Autodesk Inventor part; units mm, degrees
ref_plane "YZ Plane" through (0, 0, 0) normal (1, 0, 0) x (0, 1, 0)
ref_plane "XZ Plane" through (0, 0, 0) normal (0, 1, 0) x (-1, 0, 0)
ref_plane "XY Plane" through (0, 0, 0) normal (0, 0, 1) x (1, 0, 0)
sketch "Skizze2" plane through (0, 0, 0) normal (0, 0, 1) x (1, 0, 0)
  line L0 (-26.1954, 0) -> (26.1954, 0)
  line L1 (0, -30.2532) -> (0, 68.0422)
  line L2 (-18.5, 54) -> (-18.5, -6.7574)
  line L3 (-9.2574, -16) -> (9.2574, -16)
  line L4 (18.5, -6.7574) -> (18.5, 54)
  line L5 (18.5, 54) -> (11, 54)
  line L6 (11, 54) -> (11, 3)
  line L7 (-11, 3) -> (-11, 54)
  line L8 (-11, 54) -> (-18.5, 54)
  circle A0 centre (0, -10) radius 3.15
  circle A1 centre (-14.75, 43) radius 1.3
  circle A2 centre (-14.75, 30) radius 1.3
  circle A3 centre (-14.75, 17) radius 1.3
  circle A4 centre (-14.75, 3) radius 1.3
  circle A5 centre (14.75, 43) radius 1.3
  circle A6 centre (14.75, 30) radius 1.3
  circle A7 centre (14.75, 17) radius 1.3
  circle A8 centre (14.75, 3) radius 1.3
  line L9 (-17.6213, -8.8787) -> (-11.3787, -15.1213)
  line L10 (11.3787, -15.1213) -> (17.6213, -8.8787)
  arc A9 (-18.5, -6.7574) -> (-17.6213, -8.8787) centre (-15.5, -6.7574) ccw
  arc A10 (-11.3787, -15.1213) -> (-9.2574, -16) centre (-9.2574, -13) ccw
  arc A11 (9.2574, -16) -> (11.3787, -15.1213) centre (9.2574, -13) ccw
  line L11 (-11, 3) -> (-11, 0.2426)
  line L12 (11, 3) -> (11, 0.2426)
  line L13 (-6.7574, -4) -> (6.7574, -4)
  line L14 (-10.1213, -1.8787) -> (-8.8787, -3.1213)
  line L15 (8.8787, -3.1213) -> (10.1213, -1.8787)
  arc A12 (-11, 0.2426) -> (-10.1213, -1.8787) centre (-8, 0.2426) ccw
  arc A13 (-8.8787, -3.1213) -> (-6.7574, -4) centre (-6.7574, -1) ccw
  arc A14 (6.7574, -4) -> (8.8787, -3.1213) centre (6.7574, -1) ccw
  arc A15 (10.1213, -1.8787) -> (11, 0.2426) centre (8, 0.2426) ccw
  arc A16 (17.6213, -8.8787) -> (18.5, -6.7574) centre (15.5, -6.7574) ccw
  point P0 (0, 0)
  point P1 (-18.5, -16)
  point P2 (18.5, -16)
  point P3 (11, 0)
  point P4 (-11, 0)
  point P5 (-8, 0)
  point P6 (-11, 3)
  point P7 (8, 0)
  point P8 (11, 3)
  point P9 (-18.5, -8)
  point P10 (-10.5, -16)
  point P11 (10.5, -16)
  point P12 (18.5, -8)
  point P13 (-11, -4)
  point P14 (11, -4)
  point P15 (-11, -1)
  point P16 (-8, -4)
  point P17 (8, -4)
  point P18 (11, -1)
  dimension "d0" = 70
  dimension "d1" = 37
  dimension "d2" = 90
  dimension "d3" = 70
  dimension "d4" = 90
  dimension "d6" = 7.5
  dimension "d8" = 90
  dimension "d9" = 22
  dimension "d10" = 54
  dimension "d11" = 6.3
  dimension "d13" = 6
  dimension "d14" = 2.6
  dimension "d15" = 3.75
  dimension "d16" = 11
  dimension "d17" = 2.6
  dimension "d18" = 2.6
  dimension "d19" = 2.6
  dimension "d20" = 13
  dimension "d21" = 13
  dimension "d22" = 14
  dimension "d23" = 3.75
  dimension "d24" = 3.75
  dimension "d25" = 3.75
  dimension "d26" = 2.6
  dimension "d27" = 2.6
  dimension "d28" = 2.6
  dimension "d29" = 2.6
  dimension "d30" = 3.75
  dimension "d31" = 3
  dimension "d32" = 3
  dimension "d33" = 3
  dimension "d34" = 3
  dimension "d35" = 8
  dimension "d36" = 8
  dimension "d37" = 8
  dimension "d38" = 8
  dimension "d45" = 7
  dimension "d46" = 7
  dimension "d47" = 3
  dimension "d48" = 3
  dimension "d49" = 3
  dimension "d50" = 3
  dimension "d51" = 3
  dimension "d52" = 90
  dimension "d53" = 54
  dimension "d54" = 4
  dimension "d55" = 11
  dimension "d56" = 8
  dimension "d57" = 8
  dimension "d58" = 3
extrude "Extrusion1" add sketch "Skizze2" along normal blind 4 contours L2 L8 L7 L11 A12 L0 | L0 A12 L14 A13 L13 L1 A0 L3 A10 L9 A9 L2 | A15 L12 L6 L5 L4 L0 | L0 L4 A16 L10 A11 L3 L1 A0 L13 A14 L15 A15
equation "\"d14\" = d29"
equation "\"d17\" = d28"
equation "\"d18\" = d28"
equation "\"d19\" = d29"
equation "\"d23\" = d24"
equation "\"d24\" = d25"
equation "\"d25\" = d15"
equation "\"d26\" = d29"
equation "\"d27\" = d28"
equation "\"d28\" = d29"
equation "\"d30\" = d15"
properties part number "Part1_new1" material "Aluminium 6061"
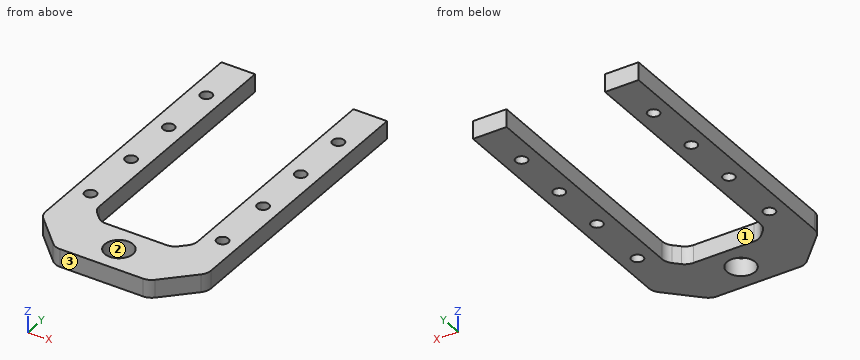
Model file for the job. Use its own axes, mm. Face numbers are marked on the shaded views. Give positions to 0.01 mm unless a question says otherwise; leave off trailing zeros. Loops run counter-clockwise (first coordinate to the right, second up) from the corner with the lowest first, then second, coordinate; pieces in that order, holes last.
1) Saw through at B-B (y = 43). Write the cut outline in (x, z).
2) Saw through at A-A (x = 0). Write the cut outline in (y, z).
3) Saw through at D-D (x = -14.75). Write the cut outline in (y, z).
4) Wall check: line 1 (X direction, y = 9.5, z = 1.2); line 2 (Y direction, x = -14.75, z = 2.4); line 3 (Y direction, x = 0, z = 0.45). Give the ranges that are in metal, low to high.
5) Flat gauge pin, fed straight in: pin 1 Ø1 at (x, z) = (-11.5, 3.5) entering from -Y. Where does the tip first touch, or does it go through?
6) Pull direction Y, two halves, no side cores. Call the marked faces 1, 2 and 3: +Y half, -Y half, draft (parallel to the pull), parting line (faces both ways), or undercut.
7) Saw through at C-C (z = 1.8). Count the separate pieces of the cut face and the enclosed holes in it, plus the area to 3 significant figures.
Answer block:
1. outline: (-18.5, 0) - (-16.05, 0) - (-16.05, 4) - (-18.5, 4) - close; (-13.45, 0) - (-11, 0) - (-11, 4) - (-13.45, 4) - close; (11, 0) - (13.45, 0) - (13.45, 4) - (11, 4) - close; (16.05, 0) - (18.5, 0) - (18.5, 4) - (16.05, 4) - close
2. outline: (-16, 0) - (-13.15, 0) - (-13.15, 4) - (-16, 4) - close; (-6.85, 0) - (-4, 0) - (-4, 4) - (-6.85, 4) - close
3. outline: (-11.75, 0) - (1.7, 0) - (1.7, 4) - (-11.75, 4) - close; (4.3, 0) - (15.7, 0) - (15.7, 4) - (4.3, 4) - close; (18.3, 0) - (28.7, 0) - (28.7, 4) - (18.3, 4) - close; (31.3, 0) - (41.7, 0) - (41.7, 4) - (31.3, 4) - close; (44.3, 0) - (54, 0) - (54, 4) - (44.3, 4) - close
4. line 1: x = -18.5 to -11, 11 to 18.5
4. line 2: y = -11.75 to 1.7, 4.3 to 15.7, 18.3 to 28.7, 31.3 to 41.7, 44.3 to 54
4. line 3: y = -16 to -13.15, -6.85 to -4
5. pin 1: stops at y = -15.44
6. face 1: +Y half
6. face 2: undercut
6. face 3: -Y half
7. separate pieces: 1
7. enclosed holes: 9
7. area: 1,190 mm2
